from build123d import *

# Parameters (mm, degrees)
SKIZZE1_R                        = 52
AUFSATZ_LINEAR_AUSTRAGEN1_DEPTH  = 3
SKIZZE1_3_R                      = 55
SKIZZE1_3_R_2                    = 52
AUFSATZ_LINEAR_AUSTRAGEN2_DEPTH  = 1.5
SCHNITT_LINEAR_AUSTRAGEN1_REACH  = 79.84
SKIZZE3_R                        = 1.6
AUFSATZ_LINEAR_AUSTRAGEN3_DEPTH  = 33
SCHNITT_LINEAR_AUSTRAGEN4_REACH  = 120.458
SCHNITT_LINEAR_START             = -4
VERRUNDUNG1_R                    = 6
SCHNITT_LINEAR_AUSTRAGEN9_DEPTH  = 6
VERRUNDUNG2_R                    = 6
VERRUNDUNG4_R                    = 6
VERRUNDUNG5_R                    = 6
VERRUNDUNG6_R                    = 2
SCHNITT_LINEAR_AUSTRAGEN10_REACH = 116.458
SKIZZE8_R                        = 1.6
SCHNITT_LINEAR_AUSTRAGEN11_REACH = 116.458
SKIZZE9_R                        = 1.6
VERRUNDUNG7_R                    = 6
SCHNITT_LINEAR_AUSTRAGEN13_REACH = 87.709
SKIZZE10_R                       = 1.6
FASE1_SIZE                       = 2


# Some blends are built 0.0001 mm under size
with BuildPart() as part:
    # Skizze1 → Aufsatz-Linear austragen1 (new body)
    with BuildSketch(Plane.XY):
        Circle(SKIZZE1_R)
    extrude(amount=AUFSATZ_LINEAR_AUSTRAGEN1_DEPTH)

    # Skizze1<3> → Aufsatz-Linear austragen2 (add)
    with BuildSketch(Plane.XY):
        Circle(SKIZZE1_3_R)
        Circle(SKIZZE1_3_R_2, mode=Mode.SUBTRACT)
    extrude(amount=AUFSATZ_LINEAR_AUSTRAGEN2_DEPTH)

    # Skizze3 → Schnitt-Linear austragen1 (cut, up to next)
    with BuildSketch(Plane.XY.offset(3), mode=Mode.PRIVATE) as schnitt_linear_austragen1_sk1:
        with Locations((5.041583425, 4.948905083)):
            Circle(SKIZZE3_R)
    schnitt_linear_austragen1_tool1 = extrude(schnitt_linear_austragen1_sk1.sketch, amount=-SCHNITT_LINEAR_AUSTRAGEN1_REACH, mode=Mode.PRIVATE) & part.part
    # Skizze3 → Schnitt-Linear austragen1 (cut, up to next)
    with BuildSketch(Plane.XY.offset(3), mode=Mode.PRIVATE) as schnitt_linear_austragen1_sk2:
        with Locations((5.275786867, 29.947808034)):
            Circle(SKIZZE3_R)
    schnitt_linear_austragen1_tool2 = extrude(schnitt_linear_austragen1_sk2.sketch, amount=-SCHNITT_LINEAR_AUSTRAGEN1_REACH, mode=Mode.PRIVATE) & part.part
    # Skizze3 → Schnitt-Linear austragen1 (cut, up to next)
    with BuildSketch(Plane.XY.offset(3), mode=Mode.PRIVATE) as schnitt_linear_austragen1_sk3:
        with Locations((-29.956880706, 5.276789902)):
            Circle(SKIZZE3_R)
    schnitt_linear_austragen1_tool3 = extrude(schnitt_linear_austragen1_sk3.sketch, amount=-SCHNITT_LINEAR_AUSTRAGEN1_REACH, mode=Mode.PRIVATE) & part.part
    add(schnitt_linear_austragen1_tool1.solids().sort_by_distance((5.041583, 4.948905, 3))[0], mode=Mode.SUBTRACT)
    add(schnitt_linear_austragen1_tool2.solids().sort_by_distance((5.275787, 29.947808, 3))[0], mode=Mode.SUBTRACT)
    add(schnitt_linear_austragen1_tool3.solids().sort_by_distance((-29.956881, 5.27679, 3))[0], mode=Mode.SUBTRACT)

    # Skizze2 → Aufsatz-Linear austragen3 (add)
    with BuildSketch(Plane.XY.offset(3)):
        Polygon((26, 21), (26, 16.2), (27.2, 16.2), (28.7, 16.2), (28.7, 15), (28.7, -24.5), (28.7, -25.7), (27.2, -25.7), (26, -25.7), (16.2, -25.7), (16.2, -26), (16.2, -27.2), (16.2, -28.7), (15, -28.7), (-24.5, -28.7), (-25.7, -28.7), (-25.7, -27.2), (-25.7, -26), (-30.5, -26), (-30.5, -33.3), (-30.5, -38.7), (-24.5, -38.7), (15, -38.7), (21, -38.7), (21, -33.3), (21, -30.5), (26, -30.5), (33.3, -30.5), (38.7, -30.5), (38.7, -24.5), (38.7, 15), (38.7, 21), (33.3, 21), align=None)
    extrude(amount=AUFSATZ_LINEAR_AUSTRAGEN3_DEPTH)

    # Skizze6 → Schnitt-Linear austragen4 (cut, up to next)
    with BuildSketch(Plane.XZ.offset(38.7).offset(SCHNITT_LINEAR_START), mode=Mode.PRIVATE) as schnitt_linear_austragen4_sk1:
        Polygon((-24.25, 3), (-23.25, 33), (13.75, 33), (14.75, 3), align=None)
    schnitt_linear_austragen4_tool1 = extrude(schnitt_linear_austragen4_sk1.sketch, amount=-SCHNITT_LINEAR_AUSTRAGEN4_REACH, mode=Mode.PRIVATE) & part.part
    add(schnitt_linear_austragen4_tool1.solids().sort_by_distance((-4.75, -34.7, 17.868421))[0], mode=Mode.SUBTRACT)

    # Verrundung1
    verrundung1_edges = [part.edges().sort_by_distance(p)[0] for p in [
        (-23.25, -31.7, 33),
        (13.75, -31.7, 33),
    ]]
    fillet(verrundung1_edges, radius=VERRUNDUNG1_R)

    # Skizze7 → Schnitt-Linear austragen9 (cut)
    with BuildSketch(Plane.ZY.offset(-28.7)):
        Polygon((33, -23.25), (33, 13.75), (3, 14.75), (3, -24.25), align=None)
    extrude(amount=-SCHNITT_LINEAR_AUSTRAGEN9_DEPTH, mode=Mode.SUBTRACT)

    # Verrundung2
    verrundung2_edges = [part.edges().sort_by_distance(p)[0] for p in [
        (31.7, -23.25, 33),
        (31.7, 13.75, 33),
    ]]
    fillet(verrundung2_edges, radius=VERRUNDUNG2_R)

    # Verrundung4
    verrundung4_edges = [part.edges().sort_by_distance(p)[0] for p in [
        (21, -30.5, 19.5),
    ]]
    fillet(verrundung4_edges, radius=VERRUNDUNG4_R)

    # Verrundung5
    # the kernel refuses this fillet: 6 mm, written as the material it takes off along each edge
    with BuildSketch(Plane(origin=(16.2, -25.7, 3), x_dir=(1, 0, 0), z_dir=(0, 0, 1))) as verrundung5_piece_1:
        with BuildLine():
            CenterArc((5.196152423, -6), VERRUNDUNG5_R, 90, 60)
            Line((0, -3), (0, 0))
            Line((0, 0), (5.196152423, 0))
        make_face()
    extrude(amount=45.990381057, mode=Mode.SUBTRACT)

    # Verrundung6
    verrundung6_edges = [part.edges().sort_by_distance(p)[0] for p in [
        (26, 21, 19.5),
        (-30.5, -26, 19.5),
    ]]
    fillet(verrundung6_edges, radius=VERRUNDUNG6_R)

    # Skizze8 → Schnitt-Linear austragen10 (cut, up to next)
    with BuildSketch(Plane.XZ.offset(38.7), mode=Mode.PRIVATE) as schnitt_linear_austragen10_sk1:
        with Locations(Location((4.75, 15, 0), (0, 0, 270))):
            Circle(SKIZZE8_R)
    schnitt_linear_austragen10_tool1 = extrude(schnitt_linear_austragen10_sk1.sketch, amount=-SCHNITT_LINEAR_AUSTRAGEN10_REACH, mode=Mode.PRIVATE) & part.part
    # Skizze8 → Schnitt-Linear austragen10 (cut, up to next)
    with BuildSketch(Plane.XZ.offset(38.7), mode=Mode.PRIVATE) as schnitt_linear_austragen10_sk2:
        with Locations(Location((-7.25, 15, 0), (0, 0, 270))):
            Circle(SKIZZE8_R)
    schnitt_linear_austragen10_tool2 = extrude(schnitt_linear_austragen10_sk2.sketch, amount=-SCHNITT_LINEAR_AUSTRAGEN10_REACH, mode=Mode.PRIVATE) & part.part
    add(schnitt_linear_austragen10_tool1.solids().sort_by_distance((4.75, -38.7, 15))[0], mode=Mode.SUBTRACT)
    add(schnitt_linear_austragen10_tool2.solids().sort_by_distance((-7.25, -38.7, 15))[0], mode=Mode.SUBTRACT)

    # Skizze9 → Schnitt-Linear austragen11 (cut, up to next)
    with BuildSketch(Plane(origin=(38.7, 0, 0), x_dir=(0, 0, -1), z_dir=(1, 0, 0)), mode=Mode.PRIVATE) as schnitt_linear_austragen11_sk1:
        with Locations((-15, -7.25)):
            Circle(SKIZZE9_R)
    schnitt_linear_austragen11_tool1 = extrude(schnitt_linear_austragen11_sk1.sketch, amount=-SCHNITT_LINEAR_AUSTRAGEN11_REACH, mode=Mode.PRIVATE) & part.part
    # Skizze9 → Schnitt-Linear austragen11 (cut, up to next)
    with BuildSketch(Plane(origin=(38.7, 0, 0), x_dir=(0, 0, -1), z_dir=(1, 0, 0)), mode=Mode.PRIVATE) as schnitt_linear_austragen11_sk2:
        with Locations((-15, 4.75)):
            Circle(SKIZZE9_R)
    schnitt_linear_austragen11_tool2 = extrude(schnitt_linear_austragen11_sk2.sketch, amount=-SCHNITT_LINEAR_AUSTRAGEN11_REACH, mode=Mode.PRIVATE) & part.part
    add(schnitt_linear_austragen11_tool1.solids().sort_by_distance((38.7, -7.25, 15))[0], mode=Mode.SUBTRACT)
    add(schnitt_linear_austragen11_tool2.solids().sort_by_distance((38.7, 4.75, 15))[0], mode=Mode.SUBTRACT)

    # Verrundung7
    verrundung7_edges = [part.edges().sort_by_distance(p)[0] for p in [
        (38.7, 21, 19.5),
        (-30.5, -38.7, 19.5),
        (21, -38.7, 19.5),
        (38.7, -30.5, 19.5),
    ]]
    fillet(verrundung7_edges, radius=VERRUNDUNG7_R)

    # Skizze10 → Schnitt-Linear austragen13 (cut, up to next)
    with BuildSketch(Plane(origin=(0, 0, 0), x_dir=(-1, 0, 0), z_dir=(0, 0, -1)), mode=Mode.PRIVATE) as schnitt_linear_austragen13_sk1:
        with Locations((35.355339059, -35.355339059)):
            Circle(SKIZZE10_R)
    schnitt_linear_austragen13_tool1 = extrude(schnitt_linear_austragen13_sk1.sketch, amount=-SCHNITT_LINEAR_AUSTRAGEN13_REACH, mode=Mode.PRIVATE) & part.part
    # Skizze10 → Schnitt-Linear austragen13 (cut, up to next)
    with BuildSketch(Plane(origin=(0, 0, 0), x_dir=(-1, 0, 0), z_dir=(0, 0, -1)), mode=Mode.PRIVATE) as schnitt_linear_austragen13_sk2:
        with Locations((-35.355339059, 35.355339059)):
            Circle(SKIZZE10_R)
    schnitt_linear_austragen13_tool2 = extrude(schnitt_linear_austragen13_sk2.sketch, amount=-SCHNITT_LINEAR_AUSTRAGEN13_REACH, mode=Mode.PRIVATE) & part.part
    add(schnitt_linear_austragen13_tool1.solids().sort_by_distance((-35.355339, -35.355339, 0))[0], mode=Mode.SUBTRACT)
    add(schnitt_linear_austragen13_tool2.solids().sort_by_distance((35.355339, 35.355339, 0))[0], mode=Mode.SUBTRACT)

    # Fase1
    fase1_edges = [part.edges().sort_by_distance(p)[0] for p in [
        (-30.5, -30.35, 36),
        (26, 17.6, 36),
        (26.585786438, 20.414213562, 36),
        (-29.914213562, -26.585786438, 36),
        (30.35, 21, 36),
        (38.7, -4.75, 36),
        (-4.44122131, -38.7, 36),
        (23.492864417, -31.631735422, 36),
        (29.85, -30.5, 36),
        (36.942640687, -28.742640687, 36),
        (19.124692969, -37.568264574, 36),
        (-28.742640687, -36.942640687, 36),
        (36.942640687, 19.242640687, 36),
        (-27.1, -26, 36),
    ]]
    chamfer(fase1_edges, length=FASE1_SIZE - 0.0001)  # a hair under: the kernel refuses the full size


solid = part.part
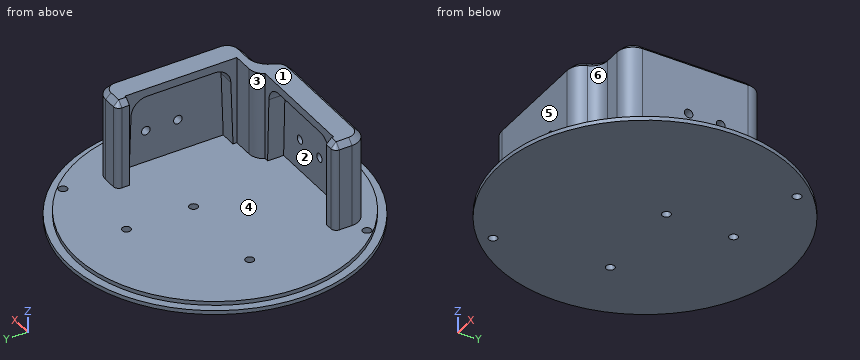
Here's how the part is built. I have some questions about the finished solid (model axes, mm). Face numbers are marked on the shaded views. A direction names the side the tool comes from. Give positions to 0.01 mm unless a question says otherwise; leave off trailing zeros. Order: outer loops, then holes, each group sorted by start corner. A loop starts at its lowest first (then second) coordinate and runs counter-clockwise, first axis right, second up. Notation, with made-up numbers: (7, -17.75) -> (30, -17.75) arc R15 ccw to (30, -10.75) -> close; hole circle Ø2 at (-8, 85). An arc over 180 degrees is marked (long way). Use a Markdown table: item, result. Add a question column.
Item 1: For the marked faces 4, 5 and 6, which set-ups out of +Z, -Z, +X, -X, +Y, -Y let a thin tool reach every point of the face, with its end or its side?
Item 2: I need wall thicknesses on line 1 (X direction, y = -37.5, z = 14.5); line 2 (X direction, y = -36.1, z = 15); line 3 (Z direction, x = 0, y = -49.5). Which ranges of each line are inside material? Lowest first, please.
Item 3: If we mould it in two halves opening along Z, with no side actions, what happens to the marked faces 1, 2 and 3? For each: pulls with the +Z half, pulls with the -Z half, needs draft (parallel to the pull), parting line crosses it, or undercut.
Item 4: Imagine slicing it at A-A on x = -7.25. Please give me the cut outline in (y, z).
Item 5: Imagine slicing it at C-C on x = 45.5. Please give me the cut outline in (y, z).
Item 6: Imagine slicing it at D-D on y = 39.5. Please give me the cut outline in (x, z), plus the area to 3 significant figures.
Item 7: Will these pins go through, and if not, where does the flat tip stop? pin 1 (5 mm diameter, centred on x = -2.5, y = 15, fed in from +Z); pin 2 (3 mm diameter, centred on x = 5.04, y = 4.95, fed in from -Z); pin 3 (4 mm diameter, centred on x = 4.75, z = 15, fed in from -Y); pin 4 (1 mm diameter, centred on y = -5, z = 31.5, fed in from +X).
Item 8: Imagine slicing it at B-B on y = 0. Please give me the cut outline in (x, z).
Data:
| question | item | result |
|---|---|---|
| 1 | face 4 | none |
| 1 | face 5 | +Z, +X, -X, -Y |
| 1 | face 6 | +Z, +X, -Y |
| 2 | line 1 | x = -28.1 to -8.77, -5.73 to 3.23, 6.27 to 19.22 |
| 2 | line 2 | x = -29.44 to -8.85, -5.65 to 3.15, 6.35 to 20.56 |
| 2 | line 3 | z = 0 to 3 |
| 3 | face 1 | pulls with the +Z half |
| 3 | face 2 | undercut |
| 3 | face 3 | needs draft |
| 4 | outline | (-54.52, 0) -> (54.52, 0) -> (54.52, 1.5) -> (51.49, 1.5) -> (51.49, 3) -> (-34.7, 3) -> (-34.7, 13.4) -> (-38.7, 13.4) -> (-38.7, 3) -> (-51.49, 3) -> (-51.49, 1.5) -> (-54.52, 1.5) -> close; (-38.7, 16.6) -> (-34.7, 16.6) -> (-34.7, 33) -> (-28.7, 33) -> (-28.7, 36) -> (-36.7, 36) -> (-38.7, 34) -> close |
| 5 | outline | (-30.9, 0) -> (30.9, 0) -> (30.9, 1.5) -> (25.17, 1.5) -> (25.17, 3) -> (-25.17, 3) -> (-25.17, 1.5) -> (-30.9, 1.5) -> close |
| 6 | outline | (-38.27, 0) -> (38.27, 0) -> (38.27, 1.5) -> (33.82, 1.5) -> (33.82, 3) -> (-33.82, 3) -> (-33.82, 1.5) -> (-38.27, 1.5) -> close |
| 6 | area | 216 mm² |
| 7 | pin 1 | stops at z = 3 |
| 7 | pin 2 | passes through |
| 7 | pin 3 | stops at y = -38.7 |
| 7 | pin 4 | stops at x = 38.7 |
| 8 | outline | (-55, 0) -> (55, 0) -> (55, 1.5) -> (52, 1.5) -> (52, 3) -> (38.7, 3) -> (38.7, 34) -> (36.7, 36) -> (28.7, 36) -> (28.7, 33) -> (34.7, 33) -> (34.7, 3) -> (-52, 3) -> (-52, 1.5) -> (-55, 1.5) -> close |
